Can you work these out from the drawing? Everything is in mm from the part's minimum corner. Coordinates: 2 decimals unless noted, no trailing zeros. Order: outer loops, then holes, each group sorted by start corner. A loop starts at its lowest first (then second) coordinate and runs counter-clockwise, first axis right, second up. Notation, with made-up numbers: (-36, 34) - (16, 34) arc R24 ccw to (16, 51) - close; hole circle Ø3 at (38.5, 60.5). An arc over 180 degrees is marked (long way). Answer as CSV lines item,"result". Start each with the question number.
Q1. Suppose I cut it at D-D (x = 2.75). Please give me the cut outline in (y, z) (3 decimals).
Q2. Thinking about a two-plate mould opening in Y: for the marked faces 1, 2, 3 and 4, which applies, released by +Y, released by -Y, zero draft, split by the parting line, or undercut?
Q3. I need wall thicknesses on line 1 (Y direction, x = 3.65, z = 4); line 2 (Y direction, x = 4.6, z = 2.5); line 3 (X direction, y = 1.5, z = 3.25). Which ranges of each line are inside material? Lowest first, please.
Q4. Suppose I cut it at B-B (z = 3.55). Please give me the cut outline in (x, y) (3 decimals), then the cut area to 3 significant figures.
Q5. Suppose I cut it at C-C (x = 4.2). Please give me the cut outline in (y, z) (3 decimals), then the cut area to 3 significant figures.
Q6. For pin 1 Ø1.5 at (y, z) = (3.5, 3.5) entering from -X; pin 2 Ø0.5 at (y, z) = (4.5, 1) entering from +X (3 decimals); pin 3 Ø1.8 at (x, z) = (2.525, 2.525) entering from +Y, each with a flat end and sliding along its axis, tell me the tip position at first contact or that it passes through.
Q7. Suppose I cut it at A-A (y = 6.5). Please give me the cut outline in (x, z) (3 decimals), then the cut area to 3 significant figures.
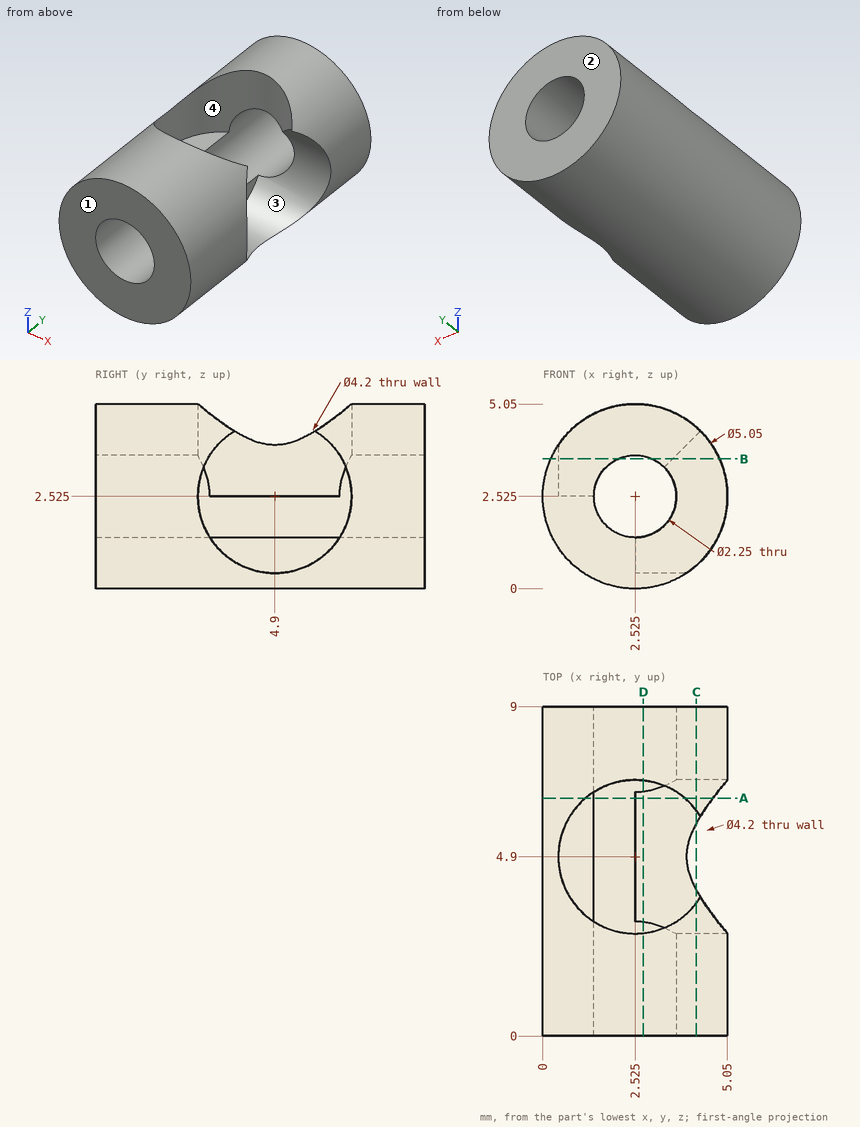
Here are the results:
1,outline,"(0, 0.01) - (9, 0.01) - (9, 1.423) - (6.687, 1.423) arc R2.1 cw to (3.113, 1.423) - (0, 1.423) - close; (0, 3.627) - (2.812, 3.627) - (2.812, 5.04) - (0, 5.04) - close; (6.988, 3.627) - (9, 3.627) - (9, 5.04) - (6.988, 5.04) - close"
2,face 1,"released by -Y"
2,face 2,"released by +Y"
2,face 3,"undercut"
2,face 4,"undercut"
3,line 1,"y = 0 to 3.13, 6.67 to 9"
3,line 2,"y = 0 to 2.8, 7 to 9"
3,line 3,"x = 0.11 to 1.66, 3.39 to 4.94"
4,outline,"(0.217, 0) - (2.061, 0) - (2.061, 2.852) arc R2.1 cw to (2.061, 6.948) - (2.061, 9) - (0.217, 9) - close; (2.989, 0) - (4.833, 0) - (4.833, 3.067) - (3.55, 3.067) arc R2.1 cw to (2.989, 2.852) - close; (2.989, 6.948) arc R2.1 cw to (3.55, 6.733) - (4.833, 6.733) - (4.833, 9) - (2.989, 9) - close"
4,area,"21.3 mm²"
5,outline,"(0, 0.636) - (3.983, 0.636) arc R2.1 cw to (3.633, 4.2) - (3.633, 4.414) - (0, 4.414) - close; (5.817, 0.636) - (9, 0.636) - (9, 4.414) - (6.167, 4.414) - (6.167, 4.2) arc R2.1 cw to start"
5,area,"20.6 mm²"
6,pin 1,"stops at x = 0.01"
6,pin 2,"stops at x = 2.525"
6,pin 3,"passes through"
7,outline,"(1.165, 2.525) - (1.165, 4.652) arc R2.525 ccw (long way) to (4.652, 1.165) - (2.525, 1.165) - (2.525, 1.4) arc R1.125 cw to (1.4, 2.525) - close; (3.885, 3.885) - (4.652, 3.885) arc R2.525 ccw to (3.885, 4.652) - close"
7,area,"7.84 mm²"
